from build123d import *

# Parameters (mm, degrees)
BOSS_EXTRUDE1_DEPTH     = 6
SKETCH3_R               = 5
BOSS_EXTRUDE2_DEPTH     = 12
SKETCH4_R               = 3
CUT_EXTRUDE1_DEPTH      = 14.4
CUT_EXTRUDE2_DEPTH      = 21.199009877
CUT_EXTRUDE2_DEPTH_BACK = 21.199009877
SKETCH5_R               = 1.5
SKETCH6_R               = 1.5
CUT_EXTRUDE3_DEPTH      = 14.4


with BuildPart() as part:
    # Sketch1 → Boss-Extrude1 (new body)
    with BuildSketch(Plane(origin=(0, 0, 0), x_dir=(1, 0, 0), z_dir=(0, 1, 0))):
        Polygon((6.92820323, 0), (3.464101615, 6), (-3.464101615, 6), (-6.92820323, 0), (-3.464101615, -6), (3.464101615, -6), align=None)
    extrude(amount=BOSS_EXTRUDE1_DEPTH)

    # Sketch3 → Boss-Extrude2 (add)
    with BuildSketch(Plane(origin=(0, 6, 0), x_dir=(1, 0, 0), z_dir=(0, 1, 0))):
        with Locations(Location((0, 0, 0), (0, 0, 270))):
            Circle(SKETCH3_R)
    extrude(amount=BOSS_EXTRUDE2_DEPTH)

    # Sketch4 → Cut-Extrude1 (cut)
    with BuildSketch(Plane(origin=(0, 18, 0), x_dir=(1, 0, 0), z_dir=(0, 1, 0))):
        with Locations(Location((0, 0, 0), (0, 0, 270))):
            Circle(SKETCH4_R)
    extrude(amount=-CUT_EXTRUDE1_DEPTH, mode=Mode.SUBTRACT)

    # Sketch5 → Cut-Extrude2 (cut, two sides: drawn at the far end of the back side and taken through both)
    with BuildSketch(Plane.XY.offset(-CUT_EXTRUDE2_DEPTH_BACK)):
        with Locations((0, 14)):
            Circle(SKETCH5_R)
    extrude(amount=CUT_EXTRUDE2_DEPTH + CUT_EXTRUDE2_DEPTH_BACK, mode=Mode.SUBTRACT)

    # Sketch6 → Cut-Extrude3 (cut)
    with BuildSketch(Plane.XZ):
        with Locations(Location((0, 0, 0), (0, 0, 270))):
            Circle(SKETCH6_R)
    extrude(amount=-CUT_EXTRUDE3_DEPTH, mode=Mode.SUBTRACT)


solid = part.part
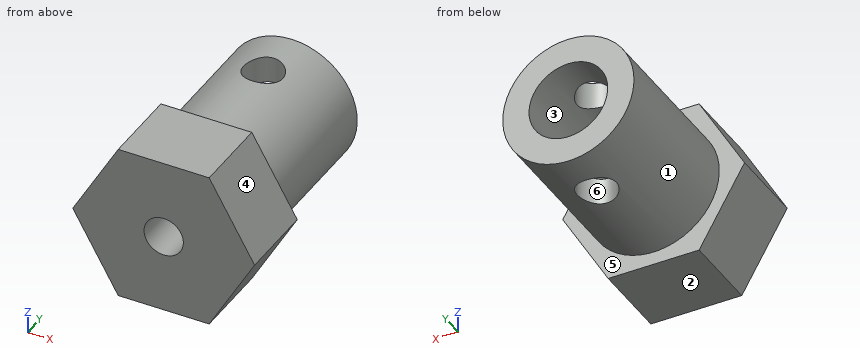
For this review, take the finished solid that the model builds, in its own axes (mm). Face numbers are marked on the shaded views. A direction names the side the tool comes from. Give positions to 0.01 mm unless a question says otherwise; leave off trailing zeros. Loops run counter-clockwise (first coordinate to the right, second up) from the corner with the lowest first, then second, coordinate; pieces in that order, holes last. Notation, with made-up numbers: (61.5, 31) -> (117.5, 31) arc R7 cw to (117.5, 38) -> close; hole circle Ø6 at (28, 72.25). An arc over 180 degrees is marked (long way). One line per question, with ' | ' between items.
1) We need section D-D (y = 14). Write out the cut boundary in (x, z).
Resolved:
outline: (-1.5, -4.77) -> (-1.5, -2.6) arc R3 cw to (-1.5, 2.6) -> (-1.5, 4.77) arc R5 ccw to start; (1.5, -4.77) arc R5 ccw to (1.5, 4.77) -> (1.5, 2.6) arc R3 cw to (1.5, -2.6) -> close
2) The part is to be moulded in two halves that separate along X. For the marked faces 3, 4, 5 and 6, say which applies: +X half, -X half, draft (parallel to the pull), parting line (faces both ways), or undercut.
Resolved:
face 3: undercut | face 4: +X half | face 5: draft | face 6: undercut
3) We need section B-B (y = 5.75). Write out the cut boundary in (x, z), plus the area to 3 significant figures.
Resolved:
outline: (-6.93, 0) -> (-3.46, -6) -> (3.46, -6) -> (6.93, 0) -> (3.46, 6) -> (-3.46, 6) -> close; hole circle Ø6 at (0, 0) | area: 96.4 mm2
4) We need section A-A (x = 0). Write out the cut boundary in (y, z), plus the area to 3 significant figures.
Resolved:
outline: (0, -6) -> (6, -6) -> (6, -5) -> (12.5, -5) -> (12.5, -3) -> (3.6, -3) -> (3.6, -1.5) -> (0, -1.5) -> close; (0, 1.5) -> (3.6, 1.5) -> (3.6, 3) -> (12.5, 3) -> (12.5, 5) -> (6, 5) -> (6, 6) -> (0, 6) -> close; (15.5, -5) -> (18, -5) -> (18, -3) -> (15.5, -3) -> close; (15.5, 3) -> (18, 3) -> (18, 5) -> (15.5, 5) -> close | area: 82.8 mm2
5) We need section C-C (z = 1.25). Write out the cut boundary in (x, y).
Resolved:
outline: (-6.21, 0) -> (-0.83, 0) -> (-0.83, 3.6) -> (-2.73, 3.6) -> (-2.73, 18) -> (-4.84, 18) -> (-4.84, 6) -> (-6.21, 6) -> close; (0.83, 0) -> (6.21, 0) -> (6.21, 6) -> (4.84, 6) -> (4.84, 18) -> (2.73, 18) -> (2.73, 3.6) -> (0.83, 3.6) -> close
6) To check wall thickness, follow probe 1 along Y at (x, z) = (5, 1.5); probe 2 along Y at (x, z) = (-0.5, -1.75); probe 3 along X at (y, z) = (14, -3.4). State the ranges of each line that lie inside material, in increasing order.
Resolved:
probe 1: y = 0 to 6 | probe 2: y = 0 to 3.6 | probe 3: x = -3.67 to -1.5, 1.5 to 3.67
7) Insertion check: pin 1 Ø3.5 at (x, z) = (0, 0) entering from +Y; pin 2 Ø2.5 at (x, y) = (0, 14) entering from +Z; pin 3 Ø1.5 at (y, z) = (7.5, -0.5) entering from -X. Each pin has a flat end and moves straight along its axis. Give the tip position at first contact, or say it passes through.
Resolved:
pin 1: stops at y = 3.6 | pin 2: passes through | pin 3: stops at x = -5
8) For the marked faces 1 and 2, list the 3-axis set-ups (+Z, -Z, +X, -X, +Y, -Y) from which the entire face can be reached by the end or side of a thin tool; tool diameter is ignored.
Resolved:
face 1: +Y | face 2: -Z, +X, -X, +Y, -Y
